The figure shows three views and two pictorial views of one solid part (mm, origin at its lowest corner). Answer the questions. Give positions to 0.01 mm unless a question says otherwise; leave off trailing zeros. Loops run counter-clockwise (first coordinate to the right, second up) from the corner with the lowest first, then second, coordinate; pieces in that order, holes last. Notation, with made-up numbers: (51, 29.5) -> (57, 29.5) arc R16 ccw to (57, 60.5) -> close; hole circle Ø2 at (-14.5, 36.5). An arc over 180 degrees is marked (long way). Answer as CSV lines item,"result". Start each with the question number.
1. Find section B-B, the plane z = 10. Give the vertices of the cut face in (x, y), and give its area (3 significant figures).
2. Find section A-A, the plane y = 45. Give the vertices of the cut face in (x, z).
3. Find section C-C, the plane y = 22. Give the vertices of the cut face in (x, z), and give its area (3 significant figures).
4. Find section D-D, the plane z = 5. Give the vertices of the cut face in (x, y).
5. Flat-ended cylindrical pins translate along their axes: pin 1 Ø1.5 at (x, y) = (50, 43.5) entering from -Z; pin 2 Ø1 at (y, z) = (26.5, 16) entering from +X; pin 3 Ø5 at (y, z) = (6, 9) entering from -X. Find the tip coordinate at first contact, or state that the pin passes through.
6. Find the intervals of material crossed by line 1 along X through (y, z) = (5.5, 8.75), in increasing order.
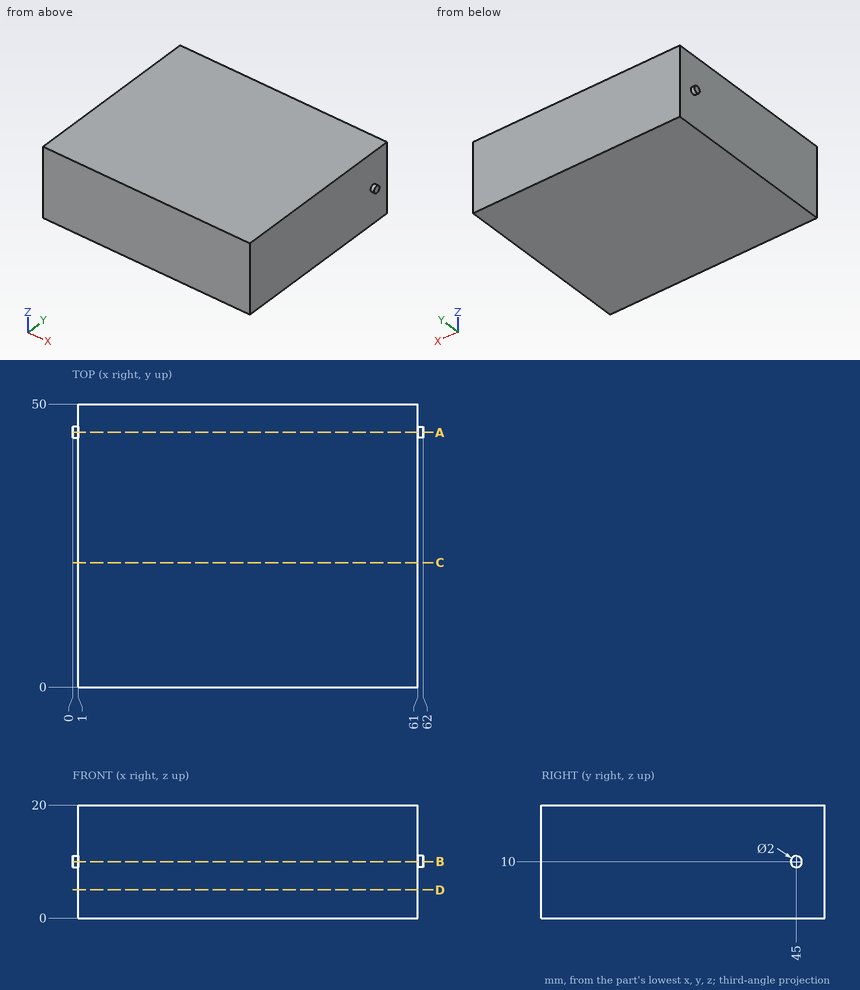
Resolved:
1,outline,"(0, 44) -> (1, 44) -> (1, 0) -> (61, 0) -> (61, 44) -> (62, 44) -> (62, 46) -> (61, 46) -> (61, 50) -> (1, 50) -> (1, 46) -> (0, 46) -> close"
1,area,"3,000 mm^2"
2,outline,"(0, 9) -> (1, 9) -> (1, 0) -> (61, 0) -> (61, 9) -> (62, 9) -> (62, 11) -> (61, 11) -> (61, 20) -> (1, 20) -> (1, 11) -> (0, 11) -> close"
3,outline,"(1, 0) -> (61, 0) -> (61, 20) -> (1, 20) -> close"
3,area,"1,200 mm^2"
4,outline,"(1, 0) -> (61, 0) -> (61, 50) -> (1, 50) -> close"
5,pin 1,"stops at z = 0"
5,pin 2,"stops at x = 61"
5,pin 3,"stops at x = 1"
6,line 1,"x = 1 to 61"
